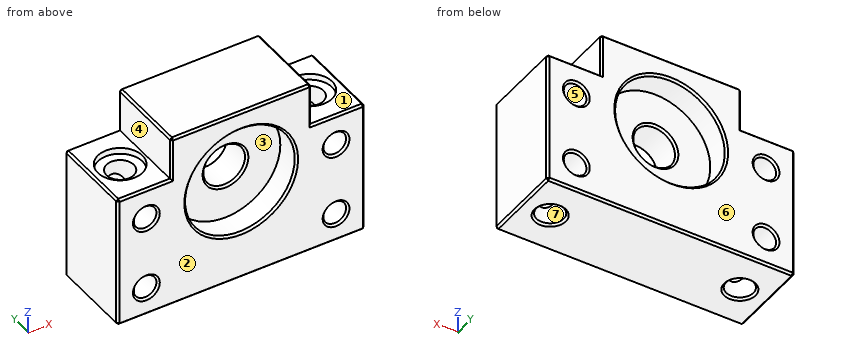
from build123d import *

# Parameters (mm, degrees)
F1_R      = 2.75
F2_DEPTH  = 20
F0_R      = 13.3
F3_DEPTH  = 20
F5_R      = 13.3
F5_R_2    = 5.05
F6_DEPTH  = 8
F7_R      = 3.3
F8_DEPTH  = 32.5
F9_R      = 5.4
F10_DEPTH = 1.5
F11_SIZE  = 0.5


with BuildPart() as f2:
    # F1 (on Front) → F2 (new body)
    with BuildSketch(Plane.XZ):
        Polygon((-17, 7.5), (-30, 7.5), (-30, -25), (30, -25), (30, 7.5), (17, 7.5), (17, 18), (-17, 18), align=None)
        with Locations((-23, -18)):
            Circle(F1_R, mode=Mode.SUBTRACT)
        with Locations((23, -18)):
            Circle(F1_R, mode=Mode.SUBTRACT)
        with Locations((-23, 0)):
            Circle(F1_R, mode=Mode.SUBTRACT)
        with Locations((23, 0)):
            Circle(F1_R, mode=Mode.SUBTRACT)
    extrude(amount=F2_DEPTH)

    # F0 (on Front) → F3 (cut, through all)
    with BuildSketch(Plane.XZ):
        Circle(F0_R)
    extrude(amount=F3_DEPTH, mode=Mode.SUBTRACT)

    # F5 (on offset) → F6 (join)
    with BuildSketch(Plane.XZ.offset(6)):
        Circle(F5_R)
        Circle(F5_R_2, mode=Mode.SUBTRACT)
    extrude(amount=F6_DEPTH)

    # F7 (on face) → F8 (cut, through all)
    with BuildSketch(Plane(origin=(0, 0, -25), x_dir=(1, 0, 0), z_dir=(0, 0, -1))):
        with Locations((-23, 10)):
            Circle(F7_R)
        with Locations((23, 10)):
            Circle(F7_R)
    extrude(amount=-F8_DEPTH, mode=Mode.SUBTRACT)

    # F9 (on face) → F10 (cut)
    with BuildSketch(Plane.XY.offset(7.5)):
        with Locations((-22.9999999999, -10)):
            Circle(F9_R)
        with Locations((23, -10)):
            Circle(F9_R)
    extrude(amount=-F10_DEPTH, mode=Mode.SUBTRACT)

    # F11
    f11_edges = [f2.edges().sort_by_distance(p)[0] for p in [
        (-17, -10, 18),
        (0, -20, 18),
        (17, -10, 18),
        (0, 0, 18),
        (-23.5, -20, 7.5),
        (-30, -10, 7.5),
        (-23.5, 0, 7.5),
        (23.5, -20, 7.5),
        (17, -20, 12.75),
        (-17, -20, 12.75),
        (-30, -20, -8.75),
        (0, -20, -25),
        (-25.75, -20, -18),
        (-25.75, -20, 0),
        (20.25, -20, 0),
        (20.25, -20, -18),
        (-13.3, -20, 0),
        (30, -20, -8.75),
        (30, -10, -25),
        (30, 0, -8.75),
        (30, -10, 7.5),
        (23.5, 0, 7.5),
        (17, 0, 12.75),
        (-5.05, -14, 0),
        (20.25, 0, 0),
        (20.25, 0, -18),
        (-25.75, 0, 0),
        (-13.3, 0, 0),
        (-30, -10, -25),
        (-30, 0, -8.75),
        (-17, 0, 12.75),
        (-25.75, 0, -18),
        (0, 0, -25),
        (-5.05, -6, 0),
        (-26.3, -10, -25),
        (19.7, -10, -25),
    ]]
    chamfer(f11_edges, length=F11_SIZE)


solid = f2.part
Read the model definition and answer for the solid it produces. Units are mm, in the model's axes. Face numbers are marked on the shaded views. A direction names the side the tool comes from. Coordinates: 2 decimals unless noted, no trailing zeros. Order: outer loops, then holes, each group sorted by start corner. A loop starts at its lowest first (then second) coordinate and runs counter-clockwise, first axis right, second up. Notation, with made-up numbers: (30, 64.25) -> (68, 64.25) arc R22 cw to (68, 70.25) -> close; hole circle Ø10 at (-18, 40.5). An arc over 180 degrees is marked (long way). Answer as a JSON object with one key per item and string values.
1) A cutting plane is placed at B-B, the plane z = -18. State how many separate pieces and enclosed holes the cut face has, plus the area to 3 significant figures.
Model answer:
{"separate pieces": "3", "enclosed holes": "0", "area": "973 mm²"}
2) The mould has two halves that part along X. Classify the marked faces 4, 5, 6 and 7: released by +X, released by -X, zero draft, split by the parting line, or undercut.
Model answer:
{"face 4": "released by -X", "face 5": "undercut", "face 6": "zero draft", "face 7": "undercut"}
3) A cutting plane is placed at A-A, the plane x = 0. Determine the outline of the cut face in (y, z), plus the area to 4 significant figures.
Model answer:
{"outline": "(-20, -24.5) -> (-19.5, -25) -> (-0.5, -25) -> (0, -24.5) -> (0, -13.8) -> (-0.5, -13.3) -> (-6, -13.3) -> (-6, -5.55) -> (-6.5, -5.05) -> (-13.5, -5.05) -> (-14, -5.55) -> (-14, -13.3) -> (-19.5, -13.3) -> (-20, -13.8) -> close; (-20, 13.8) -> (-19.5, 13.3) -> (-14, 13.3) -> (-14, 5.55) -> (-13.5, 5.05) -> (-6.5, 5.05) -> (-6, 5.55) -> (-6, 13.3) -> (-0.5, 13.3) -> (0, 13.8) -> (0, 17.5) -> (-0.5, 18) -> (-19.5, 18) -> (-20, 17.5) -> close", "area": "458.5 mm²"}
4) Each of these flat-tipped pins is pushed along its axis until it touches: pin 1 (3 mm diameter, centred on x = 5.5, z = -2, fed in from -Y); pin 2 (1 mm diameter, centred on x = 10.5, z = 2.5, fed in from +Y); pin 3 (3.5 mm diameter, centred on x = -23, z = -18, fed in from +Y); pin 4 (5.5 mm diameter, centred on x = -25, y = -11, fed in from +Z). Where does it stop, or does it pass through?
Model answer:
{"pin 1": "stops at y = -14", "pin 2": "stops at y = -6", "pin 3": "passes through", "pin 4": "stops at z = 6"}
5) A tool of negligible diameter and unlimited length cuts with its end or side. For the marked faces 1, 2 and 3, from which of +Z, -Z, +X, -X, +Y, -Y can it reach the whole face along a straight path? Write none if from no direction.
Model answer:
{"face 1": "+Z, +X, +Y, -Y", "face 2": "+Z, -Z, +X, -X, -Y", "face 3": "-Y"}
6) A cutting plane is placed at C-C, the plane y = -17. Determine the outline of the cut face in (x, z), plus the area to 3 significant figures.
Model answer:
{"outline": "(-30, -24.5) -> (-29.5, -25) -> (29.5, -25) -> (30, -24.5) -> (30, 7) -> (29.5, 7.5) -> (17, 7.5) -> (17, 17.5) -> (16.5, 18) -> (-16.5, 18) -> (-17, 17.5) -> (-17, 7.5) -> (-29.5, 7.5) -> (-30, 7) -> close; hole circle Ø5.5 at (-23, -18); hole circle Ø5.5 at (-23, 0); hole circle Ø26.6 at (0, 0); hole circle Ø5.5 at (23, -18); hole circle Ø5.5 at (23, 0)", "area": "1,660 mm²"}
7) Consider line 1 along X through (y, z) = (-15.5, -18); line 2 along X through (y, z) = (-10, -11); line 3 along X through (y, z) = (-10, -3). Determine where each line is inside the solid, lowest interval first. Write a range as from..to.
Model answer:
{"line 1": "x = -30..-25.75, -20.25..20.25, 25.75..30", "line 2": "x = -30..-26.3, -19.7..19.7, 26.3..30", "line 3": "x = -30..-26.3, -19.7..-4.06, 4.06..19.7, 26.3..30"}
